```python
from build123d import *

# Parameters (mm, degrees)
SKETCH1_W           = 120
SKETCH1_H           = 180
BOSS_EXTRUDE1_DEPTH = 5
CUT_EXTRUDE1_DEPTH  = 5
SKETCH3_R           = 1.75
CUT_EXTRUDE2_DEPTH  = 5


with BuildPart() as part:
    # Sketch1 → Boss-Extrude1 (new body)
    with BuildSketch(Plane(origin=(0, 0, 0), x_dir=(1, 0, 0), z_dir=(0, 1, 0))):
        with Locations((60, 90)):
            Rectangle(SKETCH1_W, SKETCH1_H)
    extrude(amount=BOSS_EXTRUDE1_DEPTH)

    # Sketch2 → Cut-Extrude1 (cut)
    with BuildSketch(Plane(origin=(0, 5, 0), x_dir=(1, 0, 0), z_dir=(0, 1, 0))):
        Polygon((23.35, 15), (26.65, 15), (26.65, 7.5), (27.775, 7.5), (27.775, 5), (26.65, 5), (26.65, 0), (23.35, 0), (23.35, 5), (22.225, 5), (22.225, 7.5), (23.35, 7.5), align=None)
        Polygon((76.65, 15), (76.65, 7.5), (77.775, 7.5), (77.775, 5), (76.65, 5), (76.65, 0), (73.35, 0), (73.35, 5), (72.225, 5), (72.225, 7.5), (73.35, 7.5), (73.35, 15), align=None)
        Polygon((76.65, 165), (73.35, 165), (73.35, 172.5), (72.225, 172.5), (72.225, 175), (73.35, 175), (73.35, 180), (76.65, 180), (76.65, 175), (77.775, 175), (77.775, 172.5), (76.65, 172.5), align=None)
        Polygon((23.35, 165), (23.35, 172.5), (22.225, 172.5), (22.225, 175), (23.35, 175), (23.35, 180), (26.65, 180), (26.65, 175), (27.775, 175), (27.775, 172.5), (26.65, 172.5), (26.65, 165), align=None)
    extrude(amount=-CUT_EXTRUDE1_DEPTH, mode=Mode.SUBTRACT)

    # Sketch3 → Cut-Extrude2 (cut)
    with BuildSketch(Plane(origin=(0, 5, 0), x_dir=(1, 0, 0), z_dir=(0, 1, 0))):
        with Locations(Location((25, 65, 0), (0, 0, 270))):
            Circle(SKETCH3_R)
        with Locations(Location((82, 59, 0), (0, 0, 270))):
            Circle(SKETCH3_R)
        with Locations(Location((25, 115, 0), (0, 0, 270))):
            Circle(SKETCH3_R)
        with Locations(Location((82, 121, 0), (0, 0, 270))):
            Circle(SKETCH3_R)
    extrude(amount=-CUT_EXTRUDE2_DEPTH, mode=Mode.SUBTRACT)


solid = part.part
```
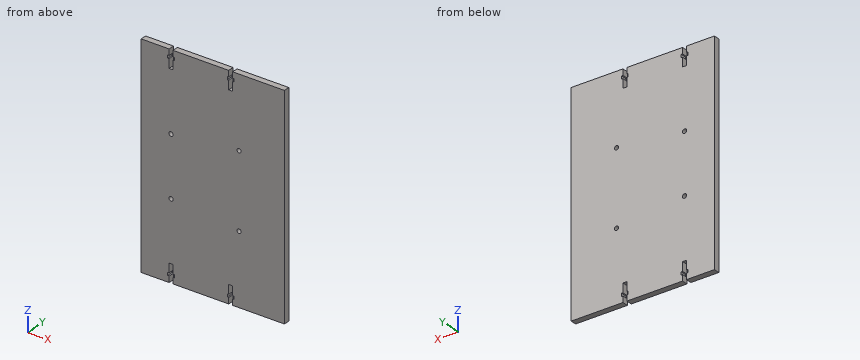
Model file for the job. Use its own axes, mm. Give positions to 0.01 mm unless a question says otherwise; leave off trailing zeros. Write each loop counter-clockwise with the first axis right and the second up, starting at its lowest first coordinate (ties: lowest second). Pieces come first, ordered by that corner, then holes. Notation, with made-up numbers: (39, 7.5) -> (95, 7.5) arc R20 ccw to (95, 32.5) -> close; hole circle Ø2 at (7.25, 58.25). An arc over 180 degrees is marked (long way). Use CSV: the item, a comma, the result in double quotes. Start each with the question number.
1) Drill centre lines: L1, parallel to Z at x = 82, y = 1.8; L2, parallel to X at y = 2.95, z = -65; L3, parallel to X at y = 3.55, z = -59. Where is each one in solid material? Low to high.
2) Cut at B-B on x = 82. List the corners of the cut face in (y, z), plus the area to 3 significant figures.
3) Cut at A-A on z = -59. List the corners of the cut face in (x, y).
Final values:
1,L1,"z = -180 to -122.75, -119.25 to -60.75, -57.25 to 0"
1,L2,"x = 0 to 23.25, 26.75 to 120"
1,L3,"x = 0 to 80.25, 83.75 to 120"
2,outline,"(0, -180) -> (5, -180) -> (5, -122.75) -> (0, -122.75) -> close; (0, -119.25) -> (5, -119.25) -> (5, -60.75) -> (0, -60.75) -> close; (0, -57.25) -> (5, -57.25) -> (5, 0) -> (0, 0) -> close"
2,area,"865 mm2"
3,outline,"(0, 0) -> (80.25, 0) -> (80.25, 5) -> (0, 5) -> close; (83.75, 0) -> (120, 0) -> (120, 5) -> (83.75, 5) -> close"
